Could you check a few things on this drawing? It's one solid part, dimensions in mm from its lowest x, y, z. Round coordinates to 2 decimals unless told otherwise and drop trailing zeros. Loops run counter-clockwise (first coordinate to the right, second up) from the corner with the lowest first, then second, coordinate; pieces in that order, holes last.
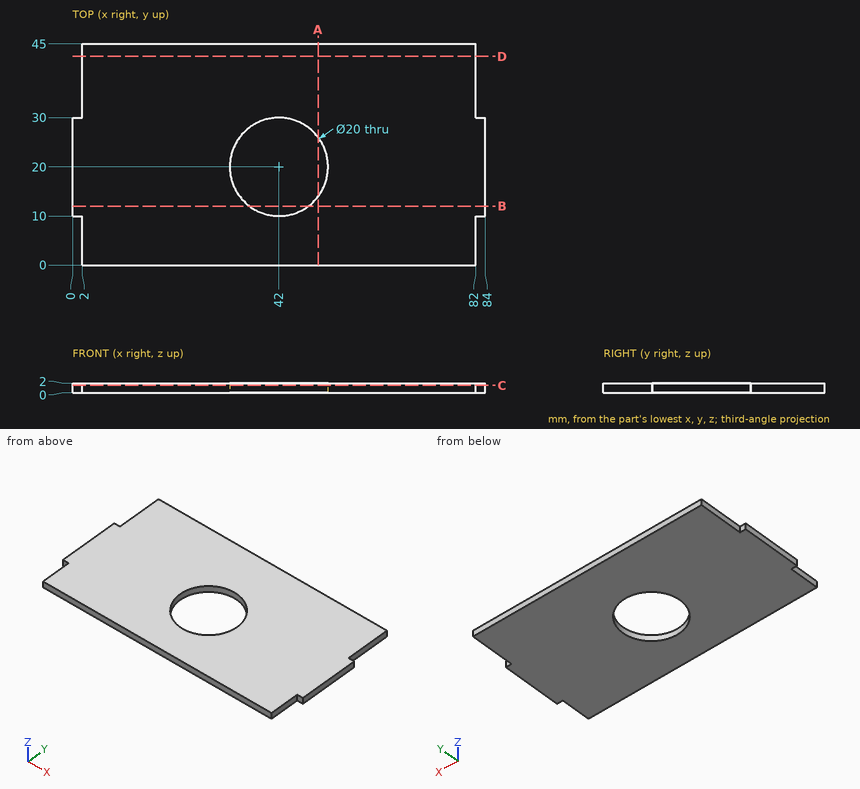
(1) Suppose I cut it at C-C (z = 1.55). Write out the boundary of the cut face in (x, y), then the cut area to 3 significant figures.
(2) Suppose I cut it at B-B (y = 12). Write out the boundary of the cut face in (x, z).
(3) Suppose I cut it at A-A (x = 50). Write out the boundary of the cut face in (y, z), then the cut area to 3 significant figures.
(4) If I drill on line 1 (Y direction, x = 42, z = 1.4); line 2 (X direction, y = 23, z = 0.35); line 3 (Y direction, x = 36.5, z = 0.5), over which ranges is the centre line in solid material (lowest first)?
(5) For pin 1 (1 mm diameter, centred on y = 7, z = 1, fed in from -X), with a flat end and sliding along its axis, tell me the tip position at first contact or that it passes through.
(6) Suppose I cut it at D-D (y = 42.5). Write out the boundary of the cut face in (x, z).
Check result:
1. outline: (0, 10) - (2, 10) - (2, 0) - (82, 0) - (82, 10) - (84, 10) - (84, 30) - (82, 30) - (82, 45) - (2, 45) - (2, 30) - (0, 30) - close; hole circle Ø20 at (42, 20)
1. area: 3,370 mm2
2. outline: (0, 0) - (36, 0) - (36, 2) - (0, 2) - close; (48, 0) - (84, 0) - (84, 2) - (48, 2) - close
3. outline: (0, 0) - (14, 0) - (14, 2) - (0, 2) - close; (26, 0) - (45, 0) - (45, 2) - (26, 2) - close
3. area: 66.0 mm2
4. line 1: y = 0 to 10, 30 to 45
4. line 2: x = 0 to 32.46, 51.54 to 84
4. line 3: y = 0 to 11.65, 28.35 to 45
5. pin 1: stops at x = 2
6. outline: (2, 0) - (82, 0) - (82, 2) - (2, 2) - close
